from build123d import *

# Parameters (mm, degrees)
SKETCH_1_W               = 60
SKETCH_1_H               = 60
EXTRUDE_1_DEPTH          = 15
EXTRUDE_START            = 15
SKETCH_2_W               = 25
SKETCH_2_H               = 25
EXTRUDE_2_DEPTH          = 40
EXTRUDE_START_2          = 12.5
EXTRUDE_3_DEPTH          = 25
CUT_EXTRUDE_START        = -12.5
SKETCH_8_R               = 6.25
CUT_EXTRUDE_5_DEPTH      = 25
CUT_EXTRUDE_6_DEPTH      = 6.25
CUT_EXTRUDE_6_DEPTH_BACK = 6.25
SKETCH_9_W               = 25
SKETCH_9_H               = 25


with BuildPart() as part:
    # 草图1 → 凸台-拉伸1 (new body)
    with BuildSketch(Plane(origin=(0, 0, 0), x_dir=(1, 0, 0), z_dir=(0, 1, 0))):
        Rectangle(SKETCH_1_W, SKETCH_1_H)
    extrude(amount=EXTRUDE_1_DEPTH)

    # 草图2 → 凸台-拉伸2 (add)
    with BuildSketch(Plane(origin=(0, 0, 0), x_dir=(1, 0, 0), z_dir=(0, 1, 0)).offset(EXTRUDE_START)):
        Rectangle(SKETCH_2_W, SKETCH_2_H)
    extrude(amount=EXTRUDE_2_DEPTH)

    # 草图6 → 凸台-拉伸3 (add)
    with BuildSketch(Plane.XY.offset(EXTRUDE_START_2)):
        with BuildLine():
            Line((-12.5, 55), (12.5, 55))
            ThreePointArc((12.5, 55), (0, 67.5), (-12.5, 55))
        make_face()
    extrude(amount=-EXTRUDE_3_DEPTH)

    # 草图8 → 切除-拉伸5 (cut)
    with BuildSketch(Plane.XY.offset(CUT_EXTRUDE_START)):
        with Locations(Location((0, 55, 0), (0, 0, 180))):
            Circle(SKETCH_8_R)
    extrude(amount=CUT_EXTRUDE_5_DEPTH, mode=Mode.SUBTRACT)

    # 草图9 → 切除-拉伸6 (cut, two sides: drawn at the far end of the back side and taken through both)
    with BuildSketch(Plane.XY.offset(-CUT_EXTRUDE_6_DEPTH_BACK)):
        with Locations((0, 55)):
            Rectangle(SKETCH_9_W, SKETCH_9_H)
    extrude(amount=CUT_EXTRUDE_6_DEPTH + CUT_EXTRUDE_6_DEPTH_BACK, mode=Mode.SUBTRACT)


solid = part.part
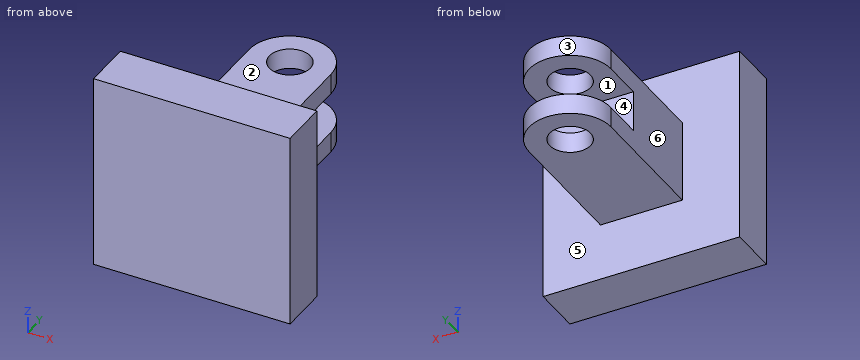
The model under review builds one solid part; all positions refer to its coordinate system, in mm. Face numbers are marked on the shaded views. A direction names the side the tool comes from. Give positions to 0.01 mm unless a question says otherwise; leave off trailing zeros. Write each loop counter-clockwise with the first axis right and the second up, starting at its lowest first coordinate (ties: lowest second). Pieces come first, ordered by that corner, then holes.
1. Add section B-B, the plane x = 0. Write out the cut boundary in (y, z), plus the area to 3 significant figures.
2. Wall thickness on L1, parallel to X at y = 55, z = -8; L2, parallel to Y at x = 0, z = 8; L3, parallel to Y at x = -15, z = -24.5: over which ranges is each line inside the solid? List them lowest first.
3. Add section C-C, the plane z = 3.5. Write out the cut boundary in (x, y), plus the area to 3 significant figures.
4. Add section D-D, the plane x = 10.5. Write out the cut boundary in (y, z), plus the area to 3 significant figures.
5. For P1, Ø1.5, axis at x = 23.5, z = 16, coming from the +Y side; P2, Ø7.5, axis at x = -3.5, y = 47, coming from the -Z side; P3, Ø14.5, axis at x = 0, y = 55, coming from the +Z side; P4, Ø10, axis at x = 0, y = 55, coming from the +Z side, all flat-tipped, find the tip position at first contact; note any pin that passes through.
6. Add section A-A, the plane y = 43.5. Write out the cut boundary in (x, z).
7. Tool access review of the marked faces 4, 5 and 6: name each direction out of +Z, -Z, +X, -X, +Y, -Y from which nothing blocks a thin tool from reaching the whole face with its end or side.
8. Draft analysis for pull direction Z (two halves, no side actions). For the marked faces 1, 2 and 3, state which applies: +Z half, -Z half, draft (parallel to the pull), parting line (faces both ways), or undercut.
Worked answers:
1. outline: (0, -30) - (15, -30) - (15, -12.5) - (48.75, -12.5) - (48.75, -6.25) - (42.5, -6.25) - (42.5, 6.25) - (48.75, 6.25) - (48.75, 12.5) - (15, 12.5) - (15, 30) - (0, 30) - close; (61.25, -12.5) - (67.5, -12.5) - (67.5, -6.25) - (61.25, -6.25) - close; (61.25, 6.25) - (67.5, 6.25) - (67.5, 12.5) - (61.25, 12.5) - close
1. area: 1,740 mm2
2. L1: x = -12.5 to -6.25, 6.25 to 12.5
2. L2: y = 0 to 48.75, 61.25 to 67.5
2. L3: y = 0 to 15
3. outline: (-30, 0) - (30, 0) - (30, 15) - (12.5, 15) - (12.5, 42.5) - (-12.5, 42.5) - (-12.5, 15) - (-30, 15) - close
3. area: 1,590 mm2
4. outline: (0, -30) - (15, -30) - (15, -12.5) - (61.78, -12.5) - (61.78, -6.25) - (42.5, -6.25) - (42.5, 6.25) - (61.78, 6.25) - (61.78, 12.5) - (15, 12.5) - (15, 30) - (0, 30) - close
4. area: 1,830 mm2
5. P1: stops at y = 15
5. P2: stops at z = -12.5
5. P3: stops at z = 12.5
5. P4: passes through
6. outline: (-12.5, -12.5) - (12.5, -12.5) - (12.5, -6.25) - (-12.5, -6.25) - close; (-12.5, 6.25) - (12.5, 6.25) - (12.5, 12.5) - (-12.5, 12.5) - close
7. face 4: +X, -X, +Y
7. face 5: +Y
7. face 6: +Z, -Z, -X, +Y
8. face 1: undercut
8. face 2: +Z half
8. face 3: draft
